Model file for the job. Use its own axes, mm. Coordinates: 2 decimals unless noted, no trailing zeros. Order: outer loops, then holes, each group sorted by start corner. A loop starts at its lowest first (then second) coordinate and runs counter-clockwise, first axis right, second up. Notation, with made-up numbers: (41.25, -0.5) - (81.25, -0.5) arc R34 ccw to (81.25, 34.5) - close; hole circle Ø10 at (-20, 9). An arc over 180 degrees is marked (long way). Put each result on its own line as item: value. Start each with the question number.
```python
from build123d import *

# Parameters (mm, degrees)
SKETCH2_R          = 1.5
CUT_EXTRUDE1_DEPTH = 7.745368782
CHAMFER1_SIZE      = 0.1


with BuildPart() as part:
    # Sketch1 → Revolve2 (revolve)
    with BuildSketch(Plane.XY):
        with BuildLine():
            Line((0, 5), (2, 5))
            ThreePointArc((2, 5), (3.201562119, 2.5), (2, 0))
            Line((2, 0), (0, 0))
            Line((0, 0), (0, 5))
        make_face()
    revolve(axis=Axis((0, 0, 0), (0, -1, 0)))

    # Sketch2 → Cut-Extrude1 (cut, through all)
    with BuildSketch(Plane(origin=(0, 5, 0), x_dir=(1, 0, 0), z_dir=(0, 1, 0))):
        with Locations(Location((0, 0, 0), (0, 0, 270))):
            Circle(SKETCH2_R)
    extrude(amount=-CUT_EXTRUDE1_DEPTH, mode=Mode.SUBTRACT)

    # Chamfer1
    chamfer1_edges = [part.edges().sort_by_distance(p)[0] for p in [
        (0, 0, -1.5),
        (0, 5, -1.5),
    ]]
    chamfer(chamfer1_edges, length=CHAMFER1_SIZE)


solid = part.part
```
Item 1: Wall check: line 1 along Z through (x, y) = (0.5, 0.95); line 2 along X through (y, z) = (1.7, 0.5); line 3 along X through (y, z) = (3.45, 0). Give the ranges that are in metal, low to high.
Item 2: Slice it at B-B, the plane z = 0. Give the cut face in (x, y), plus the area to 3 significant figures.
Item 3: Slice it at A-A, the plane x = 0. Give the cut face in (y, z).
Item 4: Slice it at D-D, the plane z = -2.25. Give the cut face in (x, y), plus the area to 3 significant figures.
Item 5: Slice it at C-C, the plane y = 2.9. Give the cut face in (x, z), plus the area to 3 significant figures.
Item 6: Flat gauge pins, fed straight in: pin 1 Ø2 at (x, z) = (-0.5, 0.5) entering from -Y; pin 2 Ø1.5 at (x, y) = (-2, 2.5) entering from -Z; pin 3 Ø2 at (x, z) = (2.5, 2) entering from -Y. Where does each tip first touch, or does it go through?
Here are the results:
1. line 1: z = -2.76 to -1.41, 1.41 to 2.76
1. line 2: x = -3.06 to -1.41, 1.41 to 3.06
1. line 3: x = -3.06 to -1.5, 1.5 to 3.06
2. outline: (-2, 0) - (-1.6, 0) - (-1.5, 0.1) - (-1.5, 4.9) - (-1.6, 5) - (-2, 5) arc R3.2 ccw to start; (1.5, 0.1) - (1.6, 0) - (2, 0) arc R3.2 ccw to (2, 5) - (1.6, 5) - (1.5, 4.9) - close
2. area: 13.3 mm^2
3. outline: (0, -2) arc R3.2 ccw to (5, -2) - (5, -1.6) - (4.9, -1.5) - (0.1, -1.5) - (0, -1.6) - close; (0, 1.6) - (0.1, 1.5) - (4.9, 1.5) - (5, 1.6) - (5, 2) arc R3.2 ccw to (0, 2) - close
4. outline: circle Ø4.56 at (0, 2.5)
4. area: 16.3 mm^2
5. outline: circle Ø6.35 at (0, 0); hole circle Ø3 at (0, 0)
5. area: 24.6 mm^2
6. pin 1: stops at y = 0
6. pin 2: stops at z = -2.95
6. pin 3: stops at y = 0.18
